For this review, use the dimensioned drawing (mm, ordinates from the lowest corner) and the shaded views. A direction names the side the tool comes from. Round coordinates to 2 decimals unless told otherwise and drop trailing zeros. Loops run counter-clockwise (first coordinate to the right, second up) from the corner with the lowest first, then second, coordinate; pieces in that order, holes last. Notation, with made-up numbers: (34.25, 81.5) -> (77.25, 81.5) arc R22 cw to (77.25, 102.5) -> close; hole circle Ø8 at (22, 51). An arc over 180 degrees is marked (long way). Write each question's results on one line, items separated by ' | '. Start each with the question number.
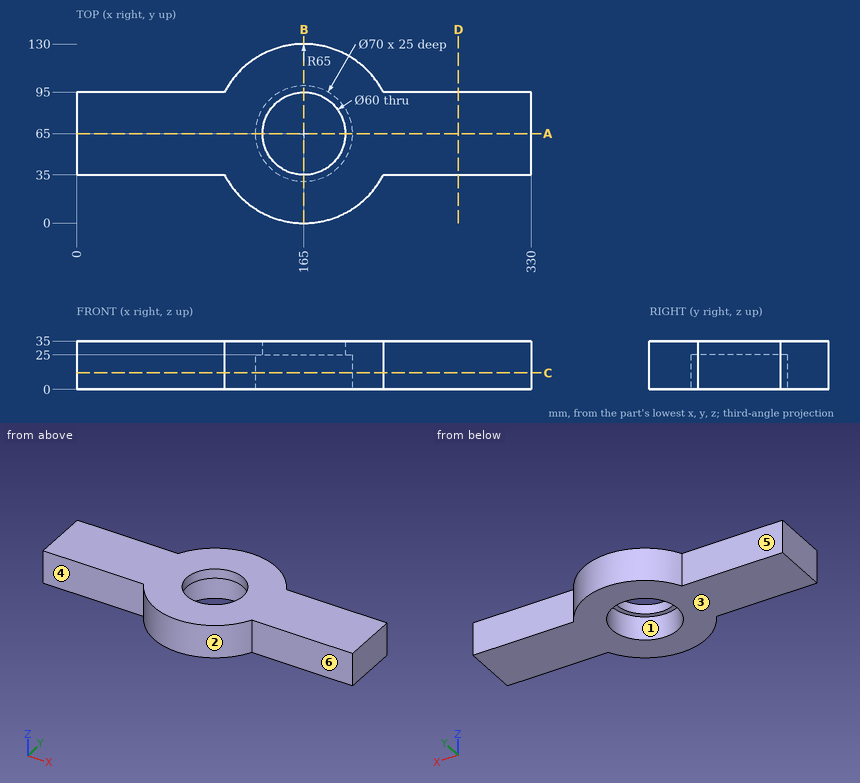
1) To check wall thickness, follow line 1 (Y direction, x = 165, z = 10.75); line 2 (Y direction, x = 165, z = 31.5); line 3 (Z direction, x = 189, y = 87). State the ranges of each line that lie inside material, in increasing order. Write a range as from..to.
2) Take a section at D-D (x = 277). Write out the cut boundary in (y, z), plus the area to 3 significant figures.
3) Take a section at A-A (y = 65). Write out the cut boundary in (x, z).
4) Take a section at C-C (z = 12). Write out the cut boundary in (x, y), plus the area to 3 significant figures.
5) Insertion check: pin 1 (5 mm diameter, centred on x = 219.5, z = 22, fed in from +Y); pin 2 (1.5 mm diameter, centred on x = 124, z = 10, fed in from +Y); pin 3 (12 mm diameter, centred on y = 101.5, z = 23, fed in from -X); pin 4 (21 mm diameter, centred on x = 162.5, y = 52.5, fed in from -Z). Each pin has a flat end and moves straight along its axis. Give the tip position at first contact, or say it passes through.
6) The part is to be moulded in two halves that separate along X. For the marked faces 1, 2 and 3, say which applies: +X half, -X half, draft (parallel to the pull), parting line (faces both ways), or undercut.
7) Take a section at B-B (x = 165). Write out the cut boundary in (y, z), plus the area to 3 significant figures.
8) For the marked faces 4, 5 and 6, list the 3-axis set-ups (+Z, -Z, +X, -X, +Y, -Y) from which the entire face can be reached by the end or side of a thin tool; tool diameter is ignored.
Geometry check:
1) line 1: y = 0..30, 100..130 | line 2: y = 0..35, 95..130 | line 3: z = 25..35
2) outline: (35, 0) -> (95, 0) -> (95, 35) -> (35, 35) -> close | area: 2,100 mm^2
3) outline: (0, 0) -> (130, 0) -> (130, 25) -> (135, 25) -> (135, 35) -> (0, 35) -> close; (195, 25) -> (200, 25) -> (200, 0) -> (330, 0) -> (330, 35) -> (195, 35) -> close
4) outline: (0, 35) -> (107.34, 35) arc R65 ccw to (222.66, 35) -> (330, 35) -> (330, 95) -> (222.66, 95) arc R65 ccw to (107.34, 95) -> (0, 95) -> close; hole circle Ø70 at (165, 65) | area: 21,700 mm^2
5) pin 1: stops at y = 104 | pin 2: stops at y = 116.04 | pin 3: stops at x = 107.6 | pin 4: passes through
6) face 1: undercut | face 2: parting line | face 3: draft
7) outline: (0, 0) -> (30, 0) -> (30, 25) -> (35, 25) -> (35, 35) -> (0, 35) -> close; (95, 25) -> (100, 25) -> (100, 0) -> (130, 0) -> (130, 35) -> (95, 35) -> close | area: 2,200 mm^2
8) face 4: +Z, -Z, -X, -Y | face 5: +Z, -Z, -X, +Y | face 6: +Z, -Z, +X, -Y
